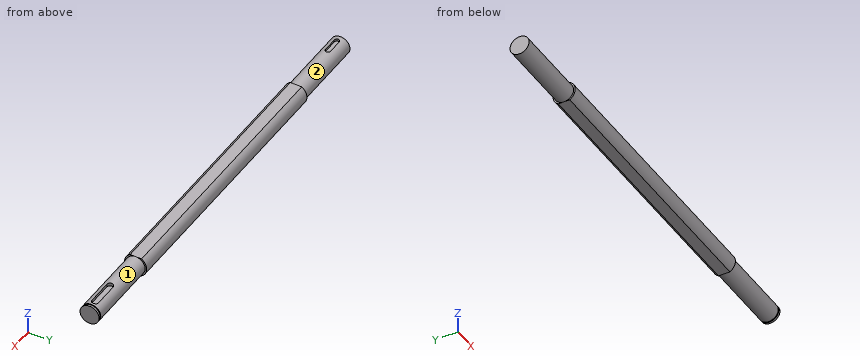
```python
from build123d import *

# Parameters (mm, degrees)
KES_EKSTR_ZYON1_DEPTH = 431
KES_EKSTR_ZYON2_DEPTH = 4
IZIM4_W               = 1.6
IZIM4_H               = 0.7
KES_EKSTR_ZYON3_DEPTH = 5


with BuildPart() as part:
    # Çizim1 → Döndür1 (revolve)
    with BuildSketch(Plane.XY, mode=Mode.PRIVATE) as d_nd_r1_sk:
        Polygon((-337.5, 0), (337.5, 0), (337.5, 15), (213.5, 15), (213.5, 17.5), (-217.5, 17.5), (-217.5, 15), (-337.5, 15), align=None)
    revolve(d_nd_r1_sk.sketch.rotate(Axis((-337.5, 0, 0), (1, 0, 0)), 90), axis=Axis((-337.5, 0, 0), (1, 0, 0)))

    # Çizim2 → Kes-Ekstrüzyon1 (cut)
    with BuildSketch(Plane.ZY.offset(217.5)):
        with BuildLine():
            Line((-14.843898339, 9.268693657), (-15.15172785, -8.756434386))
            ThreePointArc((-15.15172785, -8.756434386), (-17.49744861, 0.298817908), (-14.843898339, 9.268693657))
        make_face()
        with BuildLine():
            Line((14.843898339, 9.268693657), (15.15172785, -8.756434386))
            ThreePointArc((15.15172785, -8.756434386), (17.49744861, 0.298817908), (14.843898339, 9.268693657))
        make_face()
    extrude(amount=-KES_EKSTR_ZYON1_DEPTH, mode=Mode.SUBTRACT)

    # Çizim3 → Kes-Ekstrüzyon2 (cut)
    with BuildSketch(Plane.XY.offset(15)):
        with BuildLine():
            Line((-327.5, 4), (-303.5, 4))
            ThreePointArc((-303.5, 4), (-299.5, 0), (-303.5, -4))
            Line((-303.5, -4), (-327.5, -4))
            ThreePointArc((-327.5, -4), (-331.5, 0), (-327.5, 4))
        make_face()
    extrude(amount=-KES_EKSTR_ZYON2_DEPTH, mode=Mode.SUBTRACT)

    # Çizim4 → Kes-Döndür1 (revolve, cut)
    with BuildSketch(Plane.XY, mode=Mode.PRIVATE) as kes_d_nd_r1_sk:
        with Locations((333.7, 14.65)):
            Rectangle(IZIM4_W, IZIM4_H)
    revolve(kes_d_nd_r1_sk.sketch.rotate(Axis((337.5, 0, 0), (-1, 0, 0)), 270), axis=Axis((337.5, 0, 0), (-1, 0, 0)), mode=Mode.SUBTRACT)

    # Çizim5 → Kes-Ekstrüzyon3 (cut)
    with BuildSketch(Plane.XY.offset(15)):
        with BuildLine():
            Line((284.5, 6.07346209), (324.5, 6.07346209))
            ThreePointArc((324.5, 6.07346209), (329.5, 1.07346209), (324.5, -3.92653791))
            Line((324.5, -3.92653791), (284.5, -3.92653791))
            ThreePointArc((284.5, -3.92653791), (279.5, 1.07346209), (284.5, 6.07346209))
        make_face()
    extrude(amount=-KES_EKSTR_ZYON3_DEPTH, mode=Mode.SUBTRACT)


solid = part.part
```
Check sheet for the modelled part. Datum: model origin and axes. Units: mm. Face numbers are marked on the shaded views. A direction names the side the tool comes from. Round coordinates to 2 decimals unless told otherwise and drop trailing zeros. Order: outer loops, then holes, each group sorted by start corner. A loop starts at its lowest first (then second) coordinate and runs counter-clockwise, first axis right, second up.
1) Go/stop test with flat-tipped pins: pin 1 Ø11 at (x, y) = (317, -0.5) entering from +Z; pin 2 Ø3 at (x, z) = (-316, 12.5) entering from -Y; pin 3 Ø1.7 at (x, z) = (-320, 13.5) entering from +Y. Record where each tip stops, or that it passes through.
2) Tool access check on the marked faces 1 and 2. Record the directions out of +Z, -Z, +X, -X, +Y, -Y that give a thin tool (end or side, any length) a straight path to the whole face; none if there is none.
3) Section check B-B (x = -275). Record the boundary of the cut face in (y, z).
4) Section check C-C (x = -202). Record the boundary of the cut face in (y, z).
5) Section check A-A (z = 0). Record the boundary of the cut face in (x, y), and give its area (3 significant figures).
6) Scan lines: line 1 (X direction, y = 14, z = 5); line 2 (X direction, y = -15.5, z = -1); line 3 (Z direction, x = -8, y = 7.5). Record each from-to range of solid material in increasing order.
Result:
1. pin 1: stops at z = 14.48
1. pin 2: stops at y = -10.2
1. pin 3: stops at y = 8.06
2. face 1: +X
2. face 2: -X
3. outline: circle Ø30 at (0, 0)
4. outline: (-8.76, -15.15) - (9.27, -14.84) arc R17.5 ccw to (9.27, 14.84) - (-8.76, 15.15) arc R17.5 ccw to start
5. outline: (-337.5, -15) - (-217.5, -15) - (-217.5, -17.5) - (213.5, -17.5) - (213.5, -15) - (332.9, -15) - (332.9, -14.3) - (334.5, -14.3) - (334.5, -15) - (337.5, -15) - (337.5, 15) - (334.5, 15) - (334.5, 14.3) - (332.9, 14.3) - (332.9, 15) - (213.5, 15) - (213.5, 17.5) - (-217.5, 17.5) - (-217.5, 15) - (-337.5, 15) - close
5. area: 22,400 mm2
6. line 1: x = -337.5 to 332.9, 334.5 to 337.5
6. line 2: x = -217.5 to 213.5
6. line 3: z = -14.87 to 14.87
